```python
from build123d import *
from build123d.topology import SkipClean

# Parameters (mm, degrees)
SKETCH3_R           = 5.25
BOSS_EXTRUDE1_DEPTH = 120
BOSS_EXTRUDE4_DEPTH = 12.5
SKETCH6_R           = 3.85
BOSS_EXTRUDE5_DEPTH = 13
FILLET3_R           = 5
FILLET4_R           = 5
SKETCH7_R           = 2.65
CUT_EXTRUDE1_DEPTH  = 8
BOSS_EXTRUDE6_START = 5
BOSS_EXTRUDE6_DEPTH = 5


with BuildPart() as part:
    # Sketch3 → Boss-Extrude1 (new body)
    with BuildSketch(Plane(origin=(0, 0, 0), x_dir=(1, 0, 0), z_dir=(0, 1, 0))):
        with Locations(Location((0, 0, 0), (0, 0, 270))):
            Circle(SKETCH3_R)
    extrude(amount=BOSS_EXTRUDE1_DEPTH)

    # Sketch4 → Boss-Extrude4 (add)
    with BuildSketch(Plane.XY):
        with BuildLine():
            Line((-5.25, 0), (-5.25, -15))
            ThreePointArc((-5.25, -15), (0, -20.25), (5.25, -15))
            Line((5.25, -15), (5.25, 0))
            Line((5.25, 0), (-5.25, 0))
        make_face()
    extrude(amount=BOSS_EXTRUDE4_DEPTH)

    # Sketch6 → Boss-Extrude5 (add)
    with BuildSketch(Plane(origin=(0, 0, 0), x_dir=(-1, 0, 0), z_dir=(0, 0, -1))):
        with Locations(Location((0, -15, 0), (0, 0, 180))):
            Circle(SKETCH6_R)
    extrude(amount=BOSS_EXTRUDE5_DEPTH)

    # Fillet3
    # the kernel refuses this fillet: 5 mm, written as the material it adds along each edge
    with BuildSketch(Plane(origin=(0, 0, 0), x_dir=(0, 0, 1), z_dir=(-1, 0, 0))) as fillet3_piece_1_section:
        with BuildLine():
            CenterArc((5.25 + FILLET3_R, FILLET3_R), FILLET3_R, 180, 90)
            Line((5.25 + FILLET3_R, 0), (5.25, 0))
            Line((5.25, 0), (5.25, FILLET3_R))
        make_face()
    fillet3_piece_1 = revolve(axis=Axis((0, 0, 0), (0, 1, 0)), revolution_arc=90, mode=Mode.PRIVATE)
    fillet3_piece_1 = split(fillet3_piece_1, bisect_by=Plane(origin=(5.25, 1.168711495, 5.202443702), z_dir=(-1, 0, 0)), keep=Keep.TOP, mode=Mode.PRIVATE)
    add(fillet3_piece_1)
    with BuildSketch(Plane(origin=(0, 0, 0), x_dir=(-1, 0, 0), z_dir=(0, 0, -1))) as fillet3_piece_2_section:
        with BuildLine():
            CenterArc((5.25 + FILLET3_R, FILLET3_R), FILLET3_R, 180, 90)
            Line((5.25 + FILLET3_R, 0), (5.25, 0))
            Line((5.25, 0), (5.25, FILLET3_R))
        make_face()
    fillet3_piece_2 = revolve(axis=Axis((0, 0, 0), (0, 1, 0)), revolution_arc=90, mode=Mode.PRIVATE)
    fillet3_piece_2 = split(fillet3_piece_2, bisect_by=Plane(origin=(-5.25, 1.168711696, 5.202443347), z_dir=(1, 0, 0)), keep=Keep.TOP, mode=Mode.PRIVATE)
    add(fillet3_piece_2)

    # Fillet4
    fillet4_edges = [part.edges().sort_by_distance(p)[0] for p in [
        (5.25, -7.5, 12.5),
        (0, -20.25, 12.5),
        (-5.25, -7.5, 12.5),
    ]]
    fillet(fillet4_edges, radius=FILLET4_R)

    # Sketch7 → Cut-Extrude1 (cut)
    with BuildSketch(Plane(origin=(0, 120, 0), x_dir=(1, 0, 0), z_dir=(0, 1, 0))):
        with Locations(Location((0, 0, 0), (0, 0, 270))):
            Circle(SKETCH7_R)
    extrude(amount=-CUT_EXTRUDE1_DEPTH, mode=Mode.SUBTRACT)

    # Sketch9 → Boss-Extrude6 (add)
    with SkipClean():  # the faces are left unmerged after this step: merging them gives an invalid solid
        with BuildSketch(Plane(origin=(0, 120, 0), x_dir=(1, 0, 0), z_dir=(0, 1, 0)).offset(BOSS_EXTRUDE6_START)):
            with BuildLine():
                Line((-3.435921355, 0.666666667), (-5.153882032, 1))
                ThreePointArc((-5.153882032, 1), (0, 5.25), (5.153882032, 1))
                Line((5.153882032, 1), (3.435921355, 0.666666667))
                ThreePointArc((3.435921355, 0.666666667), (3.5, 0), (3.435921355, -0.666666667))
                Line((3.435921355, -0.666666667), (5.153882032, -1))
                ThreePointArc((5.153882032, -1), (0, -5.25), (-5.153882032, -1))
                Line((-5.153882032, -1), (-3.435921355, -0.666666667))
                ThreePointArc((-3.435921355, -0.666666667), (-3.5, 0), (-3.435921355, 0.666666667))
            make_face()
            with BuildLine():
                ThreePointArc((-2.601483311, 0.504761905), (0, 2.65), (2.601483311, 0.504761905))
                ThreePointArc((2.601483311, 0.504761905), (2.65, 0), (2.601483311, -0.504761905))
                ThreePointArc((2.601483311, -0.504761905), (0, -2.65), (-2.601483311, -0.504761905))
                ThreePointArc((-2.601483311, -0.504761905), (-2.65, 0), (-2.601483311, 0.504761905))
            make_face(mode=Mode.SUBTRACT)
        extrude(amount=-BOSS_EXTRUDE6_DEPTH)


solid = part.part
```
For this review, take the finished solid that the model builds, in its own axes (mm). A direction names the side the tool comes from. Coordinates: 2 decimals unless noted, no trailing zeros. Write each loop counter-clockwise with the first axis right and the second up, starting at its lowest first coordinate (ties: lowest second). Pieces come first, ordered by that corner, then holes. Notation, with made-up numbers: (-2.75, 14.25) - (29.25, 14.25) arc R17 cw to (29.25, 43.25) - close; hole circle Ø9 at (83.25, 40). An arc over 180 degrees is marked (long way). Answer in a Markdown table with one row per item. Add a question column.
Q1. For P1, Ø4, axis at y = 66.5, z = -7.5, coming from the +X side; P2, Ø2, axis at y = 55.5, z = 2, coming from the -X side; P3, Ø5, axis at x = 2, y = -7.5, coming from the -Z side; P4, Ø1.5, axis at x = -0.5, y = 50.5, coming from the +Z side, all flat-tipped, find the tip position at first contact; note any pin that passes through.
Q2. We need section A-A, the plane z = -11. State the section outline as (x, y) points, and give its area (3 significant figures).
Q3. For probe 1 along X at (y, z) = (116, 0); probe 2 along Y at (x, z) = (0.5, 2.75); probe 3 along X at (y, z) = (113, 1.5), list the stretches that pass through material, from the lowest coordinate up.
Q4. Tool access review of faces 1 (the flat face through (-2, 125, 2)), 2 (the cylindrical face through (-0.83, -11.24, -6.41)): name each direction out of +Z, -Z, +X, -X, +Y, -Y from which nothing blocks a thin tool from reaching the whole face with its end or side.
Q5. Draft analysis for pull direction X (two halves, no side actions). For faces 3 (the flat face through (0, 0, -2)), 4 (the cylindrical face through (-0.12, -20.25, 3.7)), 5 (the flat face through (0, 112, 0)), state which applies: +X half, -X half, draft (parallel to the pull), parting line (faces both ways), or undercut.
Q6. We need section B-B, the plane y = 38.5. State the section outline as (x, z) points.
Answer list:
| question | item | result |
|---|---|---|
| 1 | P1 | passes through |
| 1 | P2 | stops at x = -5.15 |
| 1 | P3 | stops at z = 0 |
| 1 | P4 | stops at z = 5.25 |
| 2 | outline | circle Ø7.7 at (0, -15) |
| 2 | area | 46.6 mm2 |
| 3 | probe 1 | x = -5.25 to -2.65, 2.65 to 5.25 |
| 3 | probe 2 | y = -20.23 to 125 |
| 3 | probe 3 | x = -5.03 to -2.18, 2.18 to 5.03 |
| 4 | face 1 | +Z, -Z, +X, -X, +Y |
| 4 | face 2 | -Z |
| 5 | face 3 | draft |
| 5 | face 4 | parting line |
| 5 | face 5 | undercut |
| 6 | outline | circle Ø10.5 at (0, 0) |
